from build123d import *

# Parameters (mm, degrees)
SKETCH1_R               = 7.9375
BOSS_EXTRUDE1_DEPTH     = 76.2
CUT_EXTRUDE1_DEPTH      = 128.031257511
CUT_EXTRUDE1_DEPTH_BACK = 128.031257511


with BuildPart() as part:
    # Sketch1 → Boss-Extrude1 (new body)
    with BuildSketch(Plane.XY):
        Circle(SKETCH1_R)
        Polygon((2.54, 0), (2.54, 76.2), (-2.54, 76.2), (-2.54, 0), (-2.54, -76.2), (2.54, -76.2), align=None)
        Polygon((1.27, -2.199704526), (67.261135768, 35.900295474), (64.721135768, 40.299704526), (-1.27, 2.199704526), (-67.261135768, -35.900295474), (-64.721135768, -40.299704526), align=None)
        Polygon((-1.27, -2.199704526), (64.721135768, -40.299704526), (67.261135768, -35.900295474), (1.27, 2.199704526), (-64.721135768, 40.299704526), (-67.261135768, 35.900295474), align=None)
    extrude(amount=BOSS_EXTRUDE1_DEPTH)

    # Sketch2 → Cut-Extrude1 (cut, two sides: drawn at the far end of the back side and taken through both)
    with BuildSketch(Plane.XY.offset(76.2).offset(-CUT_EXTRUDE1_DEPTH_BACK)):
        with BuildLine():
            Line((3.81, 0), (0, 3.81))
            ThreePointArc((0, 3.81), (-2.694076836, -2.694076836), (3.81, 0))
        make_face()
    extrude(amount=CUT_EXTRUDE1_DEPTH + CUT_EXTRUDE1_DEPTH_BACK, mode=Mode.SUBTRACT)


solid = part.part
Verification items for the finished model (mm, model axes). A direction names the side the tool comes from. Round coordinates to 2 decimals unless told otherwise and drop trailing zeros. Order: outer loops, then holes, each group sorted by start corner. A loop starts at its lowest first (then second) coordinate and runs counter-clockwise, first axis right, second up.
1. Release check for a two-part mould opening along X. For faces 5 (the flat face through (34.57, -22.89, 37.57)), 6 (the flat face through (-37.106, -18.49, 37.567)), 7 (the flat face through (2.54, 41, 38)), 8 (the flat face through (0, -76.2, 38)) record: +X half, -X half, draft (parallel to the pull), parting line (faces both ways), or undercut.
Final values:
face 5: undercut
face 6: -X half
face 7: undercut
face 8: draft
2. Section check B-B on x = -35. Record the cut outline in (y, z), then the cut area to 3 significant figures.
Final values:
outline: (-23.14, 0) - (-17.27, 0) - (-17.27, 76.2) - (-23.14, 76.2) - close; (17.27, 0) - (23.14, 0) - (23.14, 76.2) - (17.27, 76.2) - close
area: 894 mm2
3. Section check C-C on y = 65. Record the cut outline in (x, z).
Final values:
outline: (-2.54, 0) - (2.54, 0) - (2.54, 76.2) - (-2.54, 76.2) - close
4. Go/stop test with flat-tipped pins: P1, Ø5, axis at y = 48, z = 18.5, coming from the -X side; P2, Ø8, axis at x = -53, z = 39.5, coming from the -Y side; P3, Ø4, axis at x = -23.5, z = 58.5, coming from the +Y side. Record where each tip stops, or that it passes through.
Final values:
P1: stops at x = -2.54
P2: stops at y = -35.84
P3: stops at y = 17.66
5. Thickness scan on L1, parallel to Y at x = 0, z = 34; L2, parallel to X at y = -8.5, z = 40; L3, parallel to X at y = -21.5, z = 45. Record the ranges inside material, lowest first.
Final values:
L1: y = -76.2 to -3.81, 3.81 to 76.2
L2: x = -19.8 to -9.64, -2.54 to 2.54, 9.64 to 19.8
L3: x = -42.32 to -32.16, -2.54 to 2.54, 32.16 to 42.32
6. Section check A-A on z = 28. Record the cut outline in (x, y) (1 decimal).
Final values:
outline: (-67.3, -35.9) - (-64.7, -40.3) - (-5.2, -6) arc R7.9 ccw to (-2.5, -7.5) - (-2.5, -76.2) - (2.5, -76.2) - (2.5, -7.5) arc R7.9 ccw to (5.2, -6) - (64.7, -40.3) - (67.3, -35.9) - (7.8, -1.6) arc R7.9 ccw to (7.8, 1.6) - (67.3, 35.9) - (64.7, 40.3) - (5.2, 6) arc R7.9 ccw to (2.5, 7.5) - (2.5, 76.2) - (-2.5, 76.2) - (-2.5, 7.5) arc R7.9 ccw to (-5.2, 6) - (-64.7, 40.3) - (-67.3, 35.9) - (-7.8, 1.6) arc R7.9 ccw to (-7.8, -1.6) - close; hole (0, 3.8) arc R3.8 ccw (long way) to (3.8, 0) - close
7. Access from +Z, -Z, +X, -X, +Y, -Y to the whole of each face (thin tool, end or side, straight path). Record for faces 1 (the flat face through (-35.4, -23.37, 37.57)), 2 (the flat face through (-2.54, 42, 38)), 3 (the flat face through (37.94, -18.97, 37.57)), 4 (the flat face through (-37.94, 18.97, 37.57)).
Final values:
face 1: +Z, -Z, -Y
face 2: +Z, -Z, +Y
face 3: +Z, -Z, +X
face 4: +Z, -Z, -X
